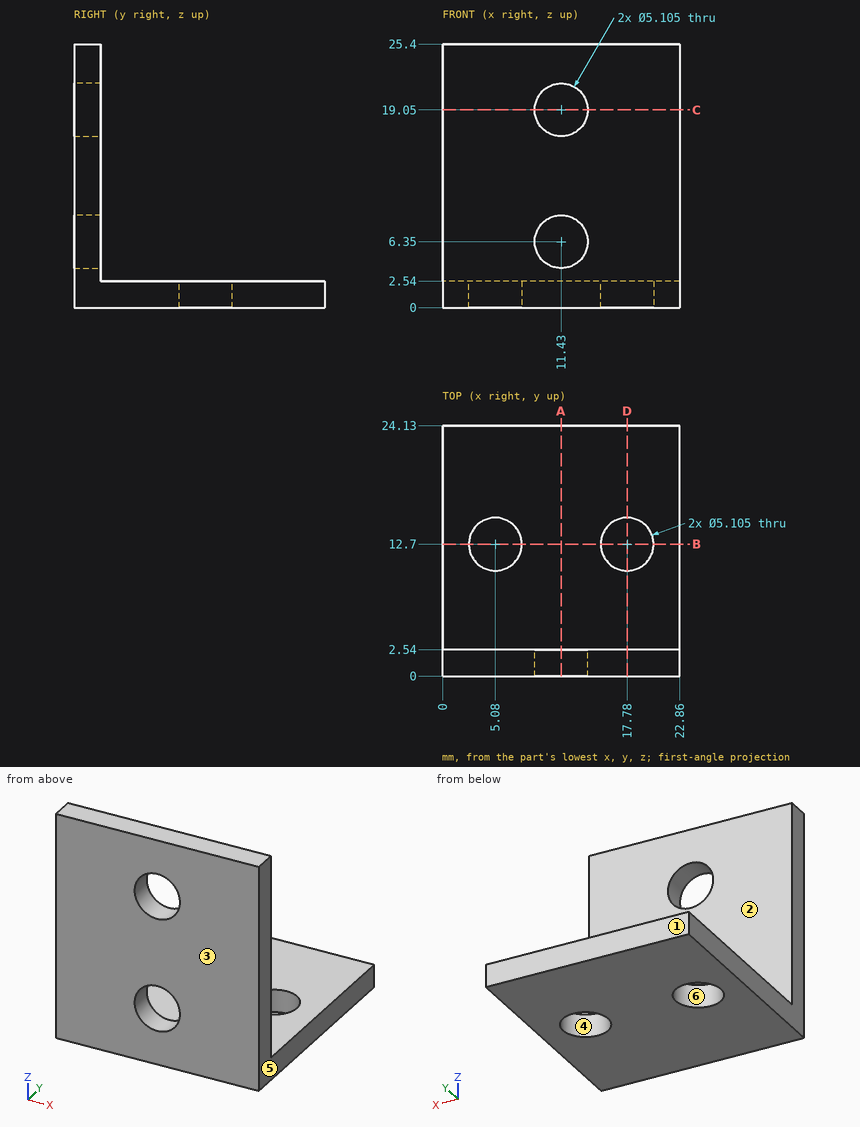
Source: three-view drawing plus pictorial views. Frame: mm from the lowest corner of the part. A direction names the side the tool comes from. Give positions to 0.01 mm unless a question says otherwise; leave off trailing zeros. Write each loop counter-clockwise with the first axis right and the second up, starting at its lowest first coordinate (ties: lowest second). Pieces come first, ordered by that corner, then holes. Notation, with made-up numbers: (77.5, 11.5) -> (108.5, 11.5) arc R21 ccw to (108.5, 49.5) -> close; hole circle Ø8 at (55, 33). An arc over 180 degrees is marked (long way). Write item = value, one per line.
Q1. Cut plane D-D on x = 17.78. Return loops of the section in (y, z), then the cut area to 3 significant figures.
Here are the results:
outline = (0, 0) -> (10.15, 0) -> (10.15, 2.54) -> (2.54, 2.54) -> (2.54, 25.4) -> (0, 25.4) -> close; (15.25, 0) -> (24.13, 0) -> (24.13, 2.54) -> (15.25, 2.54) -> close
area = 106 mm²
Q2. Reachability of the marked faces 1 and 2 from +Z, -Z, +X, -X, +Y, -Y: full face, straight path, thin tool, end or side. Return the list, or none.
Here are the results:
face_1 = +Z, -Z, +X, -X, +Y
face_2 = +Z, +X, -X, +Y
Q3. Cut plane C-C on z = 19.05. Return loops of the section in (x, y), then the cut area to 3 significant figures.
Here are the results:
outline = (0, 0) -> (8.88, 0) -> (8.88, 2.54) -> (0, 2.54) -> close; (13.98, 0) -> (22.86, 0) -> (22.86, 2.54) -> (13.98, 2.54) -> close
area = 45.1 mm²
Q4. Cut plane B-B on y = 12.7. Return loops of the section in (x, z).
Here are the results:
outline = (0, 0) -> (2.53, 0) -> (2.53, 2.54) -> (0, 2.54) -> close; (7.63, 0) -> (15.23, 0) -> (15.23, 2.54) -> (7.63, 2.54) -> close; (20.33, 0) -> (22.86, 0) -> (22.86, 2.54) -> (20.33, 2.54) -> close
Q5. First-contact query: pin 1 (8 mm diameter, centred on x = 17.78, y = 12.7, fed in from +Z); pin 2 (3 mm diameter, centred on x = 11.43, z = 6.35, fed in from +Y); pin 3 (6.5 mm diameter, centred on x = 11.43, z = 19.05, fed in from +Y). Flat tips, straight axial feed; report the tip coordinate or a pass-through.
Here are the results:
pin_1 = 2.54
pin_2 = through
pin_3 = 2.54
Q6. Line query: line 1 (Y direction, x = 17.78, z = 1.75); line 2 (X direction, y = 0.9, z = 19.05); line 3 (Z direction, x = 3.25, y = 19.5). Output: solid intervals per line, ascending. Write a range as from..to.
Here are the results:
line_1 = 0..10.15, 15.25..24.13
line_2 = 0..8.88, 13.98..22.86
line_3 = 0..2.54
Q7. Cut plane A-A on x = 11.43. Return loops of the section in (y, z).
Here are the results:
outline = (0, 0) -> (24.13, 0) -> (24.13, 2.54) -> (2.54, 2.54) -> (2.54, 3.8) -> (0, 3.8) -> close; (0, 8.9) -> (2.54, 8.9) -> (2.54, 16.5) -> (0, 16.5) -> close; (0, 21.6) -> (2.54, 21.6) -> (2.54, 25.4) -> (0, 25.4) -> close
Q8. Mould query, pull axis Y, two halves, no side actions, for the marked faces 3, 4, 5 and 6. Classes: +Y half, -Y half, draft (parallel to the pull), parting line (faces both ways), or undercut.
Here are the results:
face_3 = -Y half
face_4 = undercut
face_5 = draft
face_6 = undercut
